Part model, mm, in its own coordinate system. A direction names the side the tool comes from. Round coordinates to 2 decimals unless told otherwise and drop trailing zeros. Order: outer loops, then holes, each group sorted by start corner. A loop starts at its lowest first (then second) coordinate and runs counter-clockwise, first axis right, second up. Notation, with made-up numbers: (-15, 9.25) -> (10, 9.25) arc R32 cw to (10, 47.25) -> close; hole circle Ø6 at (-38, 47). An arc over 180 degrees is marked (long way). Answer as a JSON object with one key per item and string values. Group by question number.
Autodesk Inventor part; units mm, degrees
ref_plane "YZ Plane" through (0, 0, 0) normal (1, 0, 0) x (0, 1, 0)
ref_plane "XZ Plane" through (0, 0, 0) normal (0, 1, 0) x (-1, 0, 0)
ref_plane "XY Plane" through (0, 0, 0) normal (0, 0, 1) x (1, 0, 0)
sketch "Sketch1" plane through (0, 0, 0) normal (0, 0, 1) x (1, 0, 0)
  circle A0 centre (0, 0) radius 50
  circle A1 centre (0, 0) radius 60
  circle A2 centre (0, 0) radius 70
  circle A3 centre (-60, 0) radius 4
  circle A4 centre (-18.541, -57.0634) radius 4
  circle A5 centre (48.541, -35.2671) radius 4
  circle A6 centre (48.541, 35.2671) radius 4
  circle A7 centre (-18.541, 57.0634) radius 4
  circle A8 centre (0, 0) radius 105.3
  circle A9 centre (0, 0) radius 92.5
  circle A10 centre (0, 0) radius 99.25 construction
  line L0 (0, 0) -> (-99.25, 0) construction
  circle A11 centre (0, 0) radius 110
  circle A12 centre (-110, 0) radius 15
  circle A13 centre (0, -110) radius 15
  circle A14 centre (110, 0) radius 15
  circle A15 centre (0, 110) radius 15
  point P0 (-14.9651, -108.9773)
  point P1 (14.9651, -108.9773)
  point P2 (108.9773, -14.9651)
  point P3 (108.9773, 14.9651)
  point P4 (-14.9651, 108.9773)
  point P5 (14.9651, 108.9773)
  point P6 (-108.9773, -14.9651)
  point P7 (-108.9773, 14.9651)
  dimension "d1" = 120
  dimension "d14" = 198.5
  dimension "d22" = 220
  dimension "d0" = 100
  dimension "d2" = 140
  dimension "d3" = 8
  dimension "d6" = 360
  dimension "d12" = 210.6
  dimension "d13" = 185
  dimension "d25" = 30
  dimension "d28" = 360
extrude "Extrusion1" add sketch "Sketch1" along normal blind 2 contours A1 A5 A4 A3 A7 A6 | A2 | A9
extrude "Extrusion2" add sketch "Sketch1" along normal blind 15 contours A6 A1 | A1 A6 | A5 A1 | A1 A5 | A7 A1 | A1 A7 | A4 A1 | A1 A4 | A3 A1 | A1 A3
extrude "Extrusion3" add sketch "Sketch1" along normal blind 6 contours A8 A14 | A14 A8 A13 A12 A15 | A15 A8 | A8 A13 | A12 A8
extrude "Extrusion4" add sketch "Sketch1" along normal blind 12 contours A8 A14 A11 | A8 A15 A11 A14 | A14 A11 A13 A8 | A8 A15 A11 | A14 A11 | A13 A11 A8 | A8 A12 A11 A15 | A11 A15 | A13 A11 A12 A8 | A13 A11 | A8 A12 A11 | A11 A12
fillet "Fillet1" radius 5 4 edges at (-125, 0, 12) (0, -125, 12) (125, 0, 12) (0, 125, 12)
extrude "Extrusion5" add sketch "Sketch1" along normal blind 25 contours A8 A14 A11 | A8 A15 A11 A14 | A14 A11 A13 A8 | A8 A15 A11 | A13 A11 A8 | A8 A12 A11 A15 | A13 A11 A12 A8 | A8 A12 A11
properties part number "GroundPlate_Aperatus"
Q1. Two-plate mould, pull along X, no slides. Class faces 1 (the flat face through (40, -40, 2)), 2 (the flat face through (114, 0, 12)), 3 (the cylindrical face through (0, -125, 3)): +X half, -X half, draft (parallel to the pull), parting line (faces both ways), or undercut.
Q2. Which spindle directions (+Z, -Z, +X, -X, +Y, -Y) get a long thin tool onto all of the face, cutting with end or side? Do faces 4 (the flat face through (-19, 57, 15)), 5 (the flat face through (54, 2, 0)). Say none if no direction does.
Q3. Band-saw the part on D-D (x = -60). List the corners of the cut face in (y, z), plus the area to 3 significant figures.
Q4. Drop flat-ended pins along their axis: pin 1 Ø12 at (y, z) = (-14.5, 6.5) entering from -X; pin 2 Ø9 at (x, y) = (49, -35.5) entering from +Z; pin 3 Ø6 at (x, z) = (-20.5, 18) entering from +Y; pin 4 Ø5 at (x, y) = (-48.5, -81.5) entering from -Z. Give the stop position or say it passes through.
Q5. Wall check: line 1 (X direction, y = 0, z = 14.5); line 2 (Y direction, x = 0, z = 1.6); line 3 (Y direction, x = 45.5, z = 5). Give the ranges that are in metal, low to high. Write a range as [from, to].
Q6. Band-saw the part on B-B (x = 30.5). List the corners of the cut face in (y, z).
Q7. Band-saw the part on C-C (z = 19.5). List the corners of the cut face in (x, y).
Q8. Band-saw the part on A-A (y = 0). List the corners of the cut face in (x, z).
Completed:
{
 "1": {"face 1": "undercut", "face 2": "draft", "face 3": "parting line"},
 "2": {"face 4": "+Z", "face 5": "-Z, +X, -X, +Y, -Y"},
 "3": {"outline": "(-92.2, 0) -> (92.2, 0) -> (92.2, 25) -> (86.53, 25) -> (86.53, 6) -> (70.4, 6) -> (70.4, 2) -> (4, 2) -> (4, 15) -> (-4, 15) -> (-4, 2) -> (-70.4, 2) -> (-70.4, 6) -> (-86.53, 6) -> (-86.53, 25) -> (-92.2, 25) -> close", "area": "862 mm2"},
 "4": {"pin 1": "x = -122.36", "pin 2": "z = 15", "pin 3": "y = 108.6", "pin 4": "z = 0"},
 "5": {"line 1": "[-110, -105.3], [-64, -56], [105.3, 110]", "line 2": "[-125, -50], [50, 125]", "line 3": "[-100.15, -80.54], [-37.87, -32.67], [32.67, 37.87], [80.54, 100.15]"},
 "6": {"outline": "(-105.69, 0) -> (-39.62, 0) -> (-39.62, 2) -> (-87.33, 2) -> (-87.33, 6) -> (-100.79, 6) -> (-100.79, 25) -> (-105.69, 25) -> close; (39.62, 0) -> (105.69, 0) -> (105.69, 25) -> (100.79, 25) -> (100.79, 6) -> (87.33, 6) -> (87.33, 2) -> (39.62, 2) -> close"},
 "7": {"outline": "circle Ø220 at (0, 0); hole circle Ø210.6 at (0, 0)"},
 "8": {"outline": "(-125, 0) -> (-50, 0) -> (-50, 2) -> (-56, 2) -> (-56, 15) -> (-64, 15) -> (-64, 2) -> (-92.5, 2) -> (-92.5, 6) -> (-105.3, 6) -> (-105.3, 25) -> (-110, 25) -> (-110, 12) -> (-120, 12) arc R5 ccw to (-125, 7) -> close; (50, 0) -> (125, 0) -> (125, 7) arc R5 ccw to (120, 12) -> (110, 12) -> (110, 25) -> (105.3, 25) -> (105.3, 6) -> (92.5, 6) -> (92.5, 2) -> (50, 2) -> close"}
}
